Part print with two shaded views. Sizes in mm from the minimum x, y, z corner. A direction names the side the tool comes from. Give positions to 0.01 mm unless a question says otherwise; leave off trailing zeros. Order: outer loops, then holes, each group sorted by start corner. A loop starts at its lowest first (then second) coordinate and runs counter-clockwise, first axis right, second up. Notation, with made-up numbers: (67, 81.25) -> (91, 81.25) arc R29 ccw to (91, 113.25) -> close; hole circle Ø8 at (-18.75, 4.25). An arc over 180 degrees is marked (long way). Write item = value, one per line. Start each with the question number.
Item 1: Band-saw the part on C-C on z = 8.75. Write the cut outline in (x, y).
Item 2: Band-saw the part on B-B on x = 10. Write the cut outline in (y, z), plus the area to 3 significant figures.
Item 3: Pull direction Y, two halves, no side cores. Call the marked faces 5, 6 and 7: +Y half, -Y half, draft (parallel to the pull), parting line (faces both ways), or undercut.
Item 4: Drill centre lines: line 1 along Z through (x, y) = (12.75, 1); line 2 along X through (y, z) = (4.5, 1.25); line 3 along Z through (x, y) = (1.25, 9.5). Where is each one in solid material? Low to high.
Item 5: Tool access for the marked faces 1, 2, 3 and 4: list every direction of +Z, -Z, +X, -X, +Y, -Y with a clear straight run to the whole face (end or side of a thin tool).
Item 6: Band-saw the part on D-D on y = 3.25. Write the cut outline in (x, z).
Item 7: Band-saw the part on A-A on y = 10. Write the cut outline in (x, z), plus the area to 3 significant figures.
Item 8: Flat gauge pins, fed straight in: P1, Ø3, axis at y = 4.5, z = 2, coming from the +X side; P2, Ø1, axis at y = 6, z = 8.5, coming from the +X side; P3, Ø4, axis at x = 4.5, z = 8.5, coming from the +Y side. Where does each tip first touch, or does it go through?
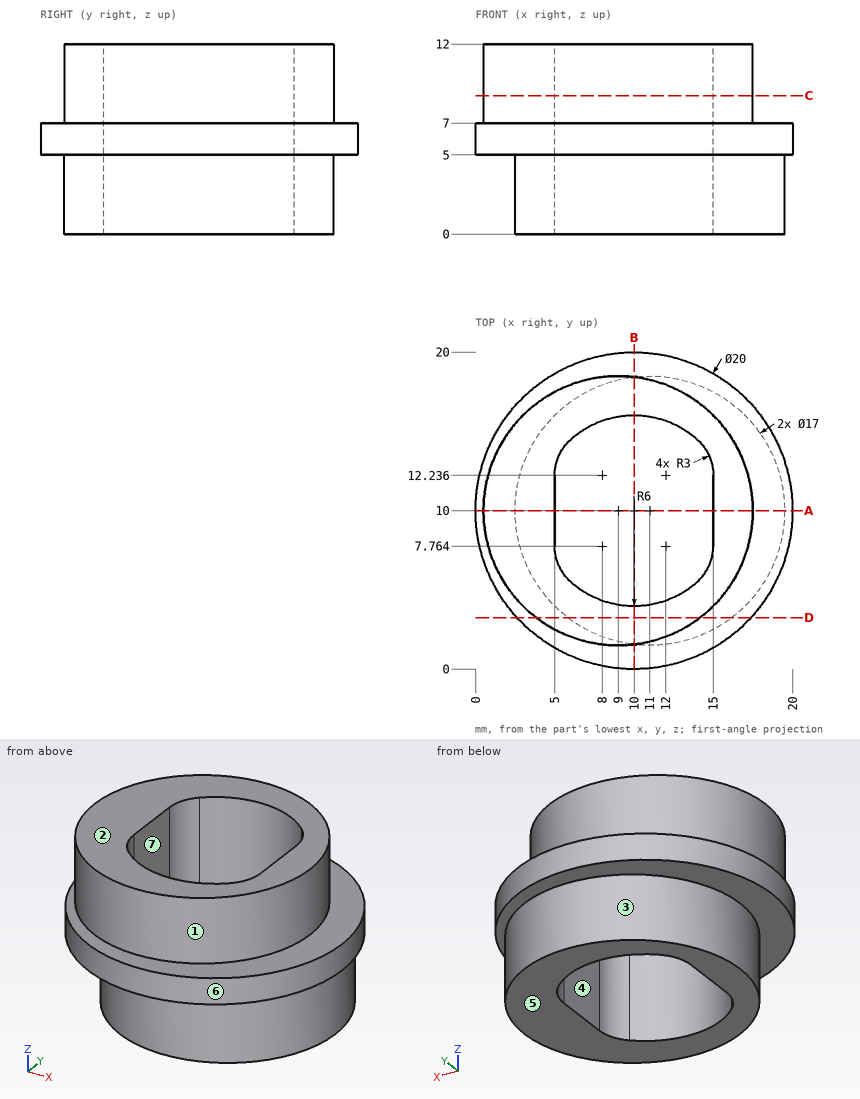
Values found:
q1.outline = circle Ø17 at (9, 10); hole (5, 7.76) arc R3 ccw to (6, 5.53) arc R6 ccw to (14, 5.53) arc R3 ccw to (15, 7.76) -> (15, 12.24) arc R3 ccw to (14, 14.47) arc R6 ccw to (6, 14.47) arc R3 ccw to (5, 12.24) -> close
q2.outline = (0, 5) -> (1.56, 5) -> (1.56, 0) -> (4, 0) -> (4, 12) -> (1.56, 12) -> (1.56, 7) -> (0, 7) -> close; (16, 0) -> (18.44, 0) -> (18.44, 5) -> (20, 5) -> (20, 7) -> (18.44, 7) -> (18.44, 12) -> (16, 12) -> close
q2.area = 64.8 mm^2
q3.face_5 = draft
q3.face_6 = parting line
q3.face_7 = undercut
q4.line_1 = 5 to 7
q4.line_2 = 4.52 to 7.6, 12.4 to 17.48
q4.line_3 = 5 to 12
q5.face_1 = +Z
q5.face_2 = +Z, +X, -X, +Y, -Y
q5.face_3 = -Z
q5.face_4 = +Z, -Z
q6.outline = (2.62, 5) -> (5.83, 5) -> (5.83, 0) -> (16.17, 0) -> (16.17, 5) -> (17.38, 5) -> (17.38, 7) -> (14.17, 7) -> (14.17, 12) -> (3.83, 12) -> (3.83, 7) -> (2.62, 7) -> close
q7.outline = (0, 5) -> (2.5, 5) -> (2.5, 0) -> (5, 0) -> (5, 12) -> (0.5, 12) -> (0.5, 7) -> (0, 7) -> close; (15, 0) -> (19.5, 0) -> (19.5, 5) -> (20, 5) -> (20, 7) -> (17.5, 7) -> (17.5, 12) -> (15, 12) -> close
q7.area = 90.0 mm^2
q8.P1 = 18.5
q8.P2 = 16.75
q8.P3 = 19.09
